from build123d import *

# Parameters (mm, degrees)
F0_R     = 35.56
F1_DEPTH = 3.175
F3_D     = 3.4544
F3_DEPTH = 11.43
F3_TIP   = 1.0378064612
F5_DEPTH = 3.176


with BuildPart() as f1:
    # F0 (on Top) → F1 (new body)
    with BuildSketch(Plane.XY):
        Circle(F0_R)
    extrude(amount=F1_DEPTH)

    # F3
    with Locations(Plane.XY.offset(3.175)):
        with Locations((-28.575, 0), (0, 28.575), (28.575, 0), (0, -28.575)):
            Hole(F3_D / 2, depth=F3_DEPTH)
            with Locations((0, 0, -(F3_DEPTH + F3_TIP / 2))):  # 118° drill point
                Cone(0, F3_D / 2, F3_TIP, mode=Mode.SUBTRACT)

    # F4 (on face) → F5 (cut, through all)
    with BuildSketch(Plane.XY.offset(3.175)):
        with BuildLine():
            ThreePointArc((-5.2927964553, -30.0169403118), (-21.5526146906, -21.5526146906), (-30.0169403118, -5.2927964553))
            Line((-30.0169403118, -5.2927964553), (-35.0197636971, -6.1749291978))
            ThreePointArc((-35.0197636971, -6.1749291978), (-25.144717139, -25.144717139), (-6.1749291978, -35.0197636971))
            Line((-6.1749291978, -35.0197636971), (-5.2927964553, -30.0169403118))
        make_face()
    extrude(amount=-F5_DEPTH, mode=Mode.SUBTRACT)


solid = f1.part
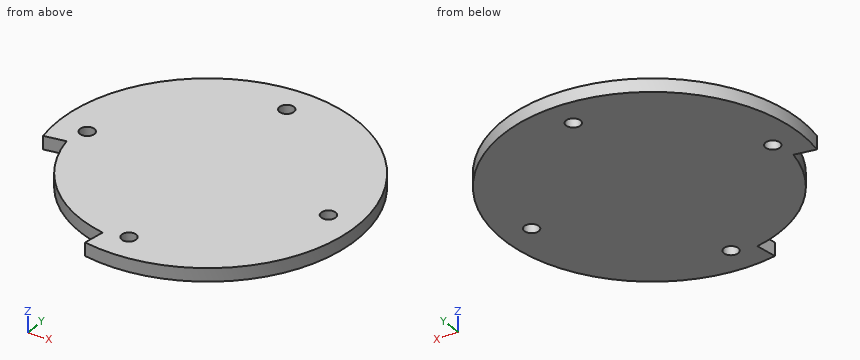
Work out the finished part from the listing and answer in its coordinate system (mm). Give positions to 0.01 mm unless a question says otherwise; leave off trailing zeros. Loops run counter-clockwise (first coordinate to the right, second up) from the corner with the lowest first, then second, coordinate; pieces in that order, holes last. Notation, with made-up numbers: M 42,18 L 86,18 A18 cw 86,51 Z; hole C -17,55.25 d9. An arc over 180 degrees is marked long. Use CSV: the item, a comma, the result in double quotes.
1) Find section C-C on z = 1.2. Write down the section's boundary in (x, y) (3 decimals), plus the area to 3 significant figures.
Answer:
outline,"M -35.02,-6.175 L -30.017,-5.293 A30.48 ccw -5.293,-30.017 L -6.175,-35.02 A35.56 ccw long Z; hole C -28.575,0 d3.454; hole C 0,-28.575 d3.454; hole C 0,28.575 d3.454; hole C 28.575,0 d3.454"
area,"3,730 mm^2"
2) Find section A-A on x = 0. Write down the section's boundary in (y, z) (3 decimals), plus the area to 3 significant figures.
Answer:
outline,"M -35.56,0 L -30.302,0 L -30.302,3.175 L -35.56,3.175 Z; M -26.848,0 L 26.848,0 L 26.848,3.175 L -26.848,3.175 Z; M 30.302,0 L 35.56,0 L 35.56,3.175 L 30.302,3.175 Z"
area,"204 mm^2"
3) Find section D-D on x = -10. Write down the section's boundary in (y, z) (3 decimals).
Answer:
outline,"M -28.793,0 L 34.125,0 L 34.125,3.175 L -28.793,3.175 Z"
4) Given P1, Ø3, axis at x = 0, y = 28.575, coming from the -Z side, flat-ended and moving along its own axis, determine where the tip first touches the part or whether it passes through.
Answer:
P1,"through"
5) Consider L1, parallel to Y at x = 0, z = 1.35; L2, parallel to X at y = 7, z = 2.35; L3, parallel to Y at x = 30.5, z = 0.65. Determine where each line is inside the solid, lowest interval first.
Answer:
L1,"-35.56 to -30.3, -26.85 to 26.85, 30.3 to 35.56"
L2,"-34.86 to 34.86"
L3,"-18.28 to 18.28"
